Read the model definition and answer for the solid it produces. Units are mm, in the model's axes. A direction names the side the tool comes from. Round coordinates to 2 decimals unless told otherwise and drop trailing zeros. Order: outer loops, then holes, each group sorted by start corner. A loop starts at its lowest first (then second) coordinate and runs counter-clockwise, first axis right, second up. Notation, with made-up numbers: (57, 32) -> (102, 32) arc R27 cw to (102, 69) -> close; hole circle Ø10 at (56, 27.5). An arc over 180 degrees is marked (long way). One line per item, written item: value. Start each with the question number.
1. For faces 5 (the face through (-431, 6.75, 620)), 6 (the face through (-3, 358.24, -9)), 7 (the face through (430, 8.25, -620)), 8 (the face through (305.38, 178.55, -8.86)), 9 (the face through (-430, 8.25, 620)), determine the directions among +Z, -Z, +X, -X, +Y, -Y from which every point of the face is accessible in a straight line to the end or side of a thin tool.
2. Section B-B (y = 283.5) is taken. Give the vertices of the cut face in (x, z), then the cut area to 3 significant figures.
3. Section D-D (x = -354) is taken. Give the vertices of the cut face in (y, z), then the cut area to 3 significant figures.
4. Section A-A (z = 13) is taken. Give the vertices of the cut face in (x, y), then the cut area to 3 significant figures.
5. Flat-ended cylindrical pins translate along their axes: pin 1 Ø10.5 at (x, z) = (427, -615) entering from +Y; pin 2 Ø4 at (x, z) = (-204, 104) entering from -Y; pin 3 Ø3 at (y, z) = (290.5, -207.5) entering from +X. Find the tip coordinate at first contact, or state that the pin passes through.
6. The mould has two halves that part along X. Classify faces 1 (the face through (431, 6.75, 620)), 2 (the face through (303.85, 184.2, -8.86)), 3 (the face through (-302.55, 183.45, -8.86)), 4 (the face through (3, 356.74, -9)): released by +X, released by -X, zero draft, split by the parting line, or undercut.
7. Section C-C (x = 1.5) is taken. Give the vertices of the cut face in (y, z).
8. Consider line 1 (Z direction, x = -447, y = 7); line 2 (X direction, y = 7, z = -615); line 3 (X direction, y = 7.65, z = -615). Determine where each line is inside the solid, lowest interval first.
from build123d import *

# Parameters (mm, degrees)
EXTRUDE_1_DEPTH          = 633
EXTRUDE_1_DEPTH_BACK     = 633
SHEET_START              = -633
SHEET_METAL_1_DEPTH      = 1266
SHEET_METAL_1_2_DEPTH    = 1266
SM_START                 = -633
SM_EDGE_FLANGE_1_DEPTH   = 33.75
SM_START_2               = -600
SM_EDGE_FLANGE_1_2_DEPTH = 0.75
SM_EDGE_FLANGE_1_3_DEPTH = 33
MIRROR_START             = -633
MIRROR_2_COPY_1_DEPTH    = 33.75
MIRROR_START_2           = -600
MIRROR_2_COPY_2_DEPTH    = 0.75
MIRROR_2_COPY_3_DEPTH    = 33
MIRROR_2_COPY_4_DEPTH    = 0.75
MIRROR_2_COPY_5_DEPTH    = 33
CUT_EXTRUDE_1_REACH      = 856.061
SKETCH_9_R               = 4


# Read off the part's stored shape, not the designer's step: Преобразовать-Твердое тело1, Ребро-кромка1
with BuildPart() as part:
    # Sketch 1 → Вытянуть-Тонкостенный1 (new, two sides: drawn at the far end of the back side and taken through both)
    with BuildSketch(Plane.XY.offset(-EXTRUDE_1_DEPTH_BACK)):
        Polygon((405, 6), (202.5, 356.740288533), (-202.5, 356.740288533), (-405, 6), (-406.299038106, 6.75), (-203.366025404, 358.240288533), (203.366025404, 358.240288533), (406.299038106, 6.75), align=None)
    extrude(amount=EXTRUDE_1_DEPTH + EXTRUDE_1_DEPTH_BACK)

    # Sheet Metal 1 outline → Sheet Metal 1 (cut)
    with BuildSketch(Plane.XY.offset(SHEET_START)):
        with BuildLine():
            Line((203.366025404, 358.240288533), (201.633974596, 358.240288533))
            ThreePointArc((201.633974596, 358.240288533), (203.133974596, 357.838364744), (204.232050808, 356.740288533))
            Line((204.232050808, 356.740288533), (203.366025404, 358.240288533))
        make_face()
        with BuildLine():
            ThreePointArc((-204.232050808, 356.740288533), (-203.133974596, 357.838364744), (-201.633974596, 358.240288533))
            Line((-201.633974596, 358.240288533), (-203.366025404, 358.240288533))
            Line((-203.366025404, 358.240288533), (-204.232050808, 356.740288533))
        make_face()
    extrude(amount=SHEET_METAL_1_DEPTH, mode=Mode.SUBTRACT)

    # Sheet Metal 1 2 outline → Sheet Metal 1 2 (add)
    with BuildSketch(Plane.XY.offset(SHEET_START)):
        with BuildLine():
            Line((202.5, 356.740288533), (201.633974596, 356.740288533))
            ThreePointArc((201.633974596, 356.740288533), (202.383974596, 356.539326638), (202.933012702, 355.990288533))
            Line((202.933012702, 355.990288533), (202.5, 356.740288533))
        make_face()
        with BuildLine():
            ThreePointArc((-202.933012702, 355.990288533), (-202.383974596, 356.539326638), (-201.633974596, 356.740288533))
            Line((-201.633974596, 356.740288533), (-202.5, 356.740288533))
            Line((-202.5, 356.740288533), (-202.933012702, 355.990288533))
        make_face()
    extrude(amount=SHEET_METAL_1_2_DEPTH)

    # Ребро-кромка1 outline → Ребро-кромка1 (cut)
    with BuildSketch(Plane.XY.offset(SM_START)):
        with BuildLine():
            Line((-405, 6), (-403.700961894, 8.25))
            ThreePointArc((-403.700961894, 8.25), (-404.799038106, 7.151923789), (-406.299038106, 6.75))
            Line((-406.299038106, 6.75), (-405, 6))
        make_face()
    sm_edge_flange_1 = extrude(amount=SM_EDGE_FLANGE_1_DEPTH, mode=Mode.SUBTRACT)

    # Sm Edge Flange 1 2 outline → Sm Edge Flange 1 2 (cut)
    with BuildSketch(Plane.XY.offset(SM_START_2)):
        with BuildLine():
            Line((-403.325961894, 8.899519053), (-404.625, 9.649519053))
            Line((-404.625, 9.649519053), (-406.299038106, 6.75))
            ThreePointArc((-406.299038106, 6.75), (-404.799038106, 7.151923789), (-403.700961894, 8.25))
            Line((-403.700961894, 8.25), (-403.325961894, 8.899519053))
        make_face()
    sm_edge_flange_1_2 = extrude(amount=SM_EDGE_FLANGE_1_2_DEPTH, mode=Mode.SUBTRACT)

    # Sm Edge Flange 1 3 outline → Sm Edge Flange 1 3 (add)
    with BuildSketch(Plane.XY.offset(SM_START)):
        with BuildLine():
            Line((-406.299038106, 6.75), (-405, 9))
            ThreePointArc((-405, 9), (-405.549038106, 8.450961894), (-406.299038106, 8.25))
            Line((-406.299038106, 8.25), (-454.133974596, 8.25))
            Line((-454.133974596, 8.25), (-454.133974596, 6.75))
            Line((-454.133974596, 6.75), (-406.299038106, 6.75))
        make_face()
    sm_edge_flange_1_3 = extrude(amount=SM_EDGE_FLANGE_1_3_DEPTH)

    # Зеркальное отражение1: Ребро-кромка1, Sm Edge Flange 1 2, Sm Edge Flange 1 3 across plane
    add(sm_edge_flange_1.mirror(Plane.XY), mode=Mode.SUBTRACT)
    add(sm_edge_flange_1_2.mirror(Plane.XY), mode=Mode.SUBTRACT)
    add(sm_edge_flange_1_3.mirror(Plane.XY))

    # Зеркальное отражение2: Ребро-кромка1, Sm Edge Flange 1 2, Sm Edge Flange 1 3 across plane
    add(sm_edge_flange_1.mirror(Plane(origin=(0, 0, 0), x_dir=(0, 0, 1), z_dir=(1, 0, 0))), mode=Mode.SUBTRACT)
    add(sm_edge_flange_1_2.mirror(Plane(origin=(0, 0, 0), x_dir=(0, 0, 1), z_dir=(1, 0, 0))), mode=Mode.SUBTRACT)
    add(sm_edge_flange_1_3.mirror(Plane(origin=(0, 0, 0), x_dir=(0, 0, 1), z_dir=(1, 0, 0))))

    # Зеркальное отражение2 copy 1 sketch → Зеркальное отражение2 copy 1 (cut)
    with BuildSketch(Plane(origin=(0, 0, 0), x_dir=(-1, 0, 0), z_dir=(0, 0, -1)).offset(MIRROR_START)):
        with BuildLine():
            Line((-405, 6), (-403.700961894, 8.25))
            ThreePointArc((-403.700961894, 8.25), (-404.799038106, 7.151923789), (-406.299038106, 6.75))
            Line((-406.299038106, 6.75), (-405, 6))
        make_face()
    extrude(amount=MIRROR_2_COPY_1_DEPTH, mode=Mode.SUBTRACT)

    # Зеркальное отражение2 copy 2 sketch → Зеркальное отражение2 copy 2 (cut)
    with BuildSketch(Plane(origin=(0, 0, 0), x_dir=(-1, 0, 0), z_dir=(0, 0, -1)).offset(MIRROR_START_2)):
        with BuildLine():
            Line((-403.325961894, 8.899519053), (-404.625, 9.649519053))
            Line((-404.625, 9.649519053), (-406.299038106, 6.75))
            ThreePointArc((-406.299038106, 6.75), (-404.799038106, 7.151923789), (-403.700961894, 8.25))
            Line((-403.700961894, 8.25), (-403.325961894, 8.899519053))
        make_face()
    extrude(amount=MIRROR_2_COPY_2_DEPTH, mode=Mode.SUBTRACT)

    # Зеркальное отражение2 copy 3 sketch → Зеркальное отражение2 copy 3 (add)
    with BuildSketch(Plane(origin=(0, 0, 0), x_dir=(-1, 0, 0), z_dir=(0, 0, -1)).offset(MIRROR_START)):
        with BuildLine():
            Line((-406.299038106, 6.75), (-405, 9))
            ThreePointArc((-405, 9), (-405.549038106, 8.450961894), (-406.299038106, 8.25))
            Line((-406.299038106, 8.25), (-454.133974596, 8.25))
            Line((-454.133974596, 8.25), (-454.133974596, 6.75))
            Line((-454.133974596, 6.75), (-406.299038106, 6.75))
        make_face()
    extrude(amount=MIRROR_2_COPY_3_DEPTH)

    # Зеркальное отражение2 copy 4 sketch → Зеркальное отражение2 copy 4 (cut)
    with BuildSketch(Plane(origin=(0, 0, 0), x_dir=(-1, 0, 0), z_dir=(0, 0, 1)).offset(MIRROR_START_2)):
        with BuildLine():
            Line((-403.325961894, -8.899519053), (-404.625, -9.649519053))
            Line((-404.625, -9.649519053), (-406.299038106, -6.75))
            ThreePointArc((-406.299038106, -6.75), (-404.799038106, -7.151923789), (-403.700961894, -8.25))
            Line((-403.700961894, -8.25), (-403.325961894, -8.899519053))
        make_face()
    extrude(amount=MIRROR_2_COPY_4_DEPTH, mode=Mode.SUBTRACT)

    # Зеркальное отражение2 copy 5 sketch → Зеркальное отражение2 copy 5 (add)
    with BuildSketch(Plane(origin=(0, 0, 0), x_dir=(-1, 0, 0), z_dir=(0, 0, 1)).offset(MIRROR_START)):
        with BuildLine():
            Line((-406.299038106, -6.75), (-405, -9))
            ThreePointArc((-405, -9), (-405.549038106, -8.450961894), (-406.299038106, -8.25))
            Line((-406.299038106, -8.25), (-454.133974596, -8.25))
            Line((-454.133974596, -8.25), (-454.133974596, -6.75))
            Line((-454.133974596, -6.75), (-406.299038106, -6.75))
        make_face()
    extrude(amount=MIRROR_2_COPY_5_DEPTH)

    # Эскиз9 → Вырез-Вытянуть1 (cut, up to next)
    with BuildSketch(Plane(origin=(0, 8.25, 0), x_dir=(1, 0, 0), z_dir=(0, 1, 0)), mode=Mode.PRIVATE) as cut_extrude_1_sk1:
        with Locations(Location((-447, 615, 0), (0, 0, 180))):
            Circle(SKETCH_9_R)
    cut_extrude_1_tool1 = extrude(cut_extrude_1_sk1.sketch, amount=-CUT_EXTRUDE_1_REACH, mode=Mode.PRIVATE) & part.part
    # Эскиз9 → Вырез-Вытянуть1 (cut, up to next)
    with BuildSketch(Plane(origin=(0, 8.25, 0), x_dir=(1, 0, 0), z_dir=(0, 1, 0)), mode=Mode.PRIVATE) as cut_extrude_1_sk2:
        with Locations(Location((-427, 615, 0), (0, 0, 180))):
            Circle(SKETCH_9_R)
    cut_extrude_1_tool2 = extrude(cut_extrude_1_sk2.sketch, amount=-CUT_EXTRUDE_1_REACH, mode=Mode.PRIVATE) & part.part
    # Эскиз9 → Вырез-Вытянуть1 (cut, up to next)
    with BuildSketch(Plane(origin=(0, 8.25, 0), x_dir=(1, 0, 0), z_dir=(0, 1, 0)), mode=Mode.PRIVATE) as cut_extrude_1_sk3:
        with Locations(Location((-447, -615, 0), (0, 0, 180))):
            Circle(SKETCH_9_R)
    cut_extrude_1_tool3 = extrude(cut_extrude_1_sk3.sketch, amount=-CUT_EXTRUDE_1_REACH, mode=Mode.PRIVATE) & part.part
    # Эскиз9 → Вырез-Вытянуть1 (cut, up to next)
    with BuildSketch(Plane(origin=(0, 8.25, 0), x_dir=(1, 0, 0), z_dir=(0, 1, 0)), mode=Mode.PRIVATE) as cut_extrude_1_sk4:
        with Locations(Location((-427, -615, 0), (0, 0, 180))):
            Circle(SKETCH_9_R)
    cut_extrude_1_tool4 = extrude(cut_extrude_1_sk4.sketch, amount=-CUT_EXTRUDE_1_REACH, mode=Mode.PRIVATE) & part.part
    # Эскиз9 → Вырез-Вытянуть1 (cut, up to next)
    with BuildSketch(Plane(origin=(0, 8.25, 0), x_dir=(1, 0, 0), z_dir=(0, 1, 0)), mode=Mode.PRIVATE) as cut_extrude_1_sk5:
        with Locations(Location((427, -615, 0), (0, 0, 180))):
            Circle(SKETCH_9_R)
    cut_extrude_1_tool5 = extrude(cut_extrude_1_sk5.sketch, amount=-CUT_EXTRUDE_1_REACH, mode=Mode.PRIVATE) & part.part
    # Эскиз9 → Вырез-Вытянуть1 (cut, up to next)
    with BuildSketch(Plane(origin=(0, 8.25, 0), x_dir=(1, 0, 0), z_dir=(0, 1, 0)), mode=Mode.PRIVATE) as cut_extrude_1_sk6:
        with Locations(Location((447, -615, 0), (0, 0, 180))):
            Circle(SKETCH_9_R)
    cut_extrude_1_tool6 = extrude(cut_extrude_1_sk6.sketch, amount=-CUT_EXTRUDE_1_REACH, mode=Mode.PRIVATE) & part.part
    # Эскиз9 → Вырез-Вытянуть1 (cut, up to next)
    with BuildSketch(Plane(origin=(0, 8.25, 0), x_dir=(1, 0, 0), z_dir=(0, 1, 0)), mode=Mode.PRIVATE) as cut_extrude_1_sk7:
        with Locations(Location((427, 615, 0), (0, 0, 180))):
            Circle(SKETCH_9_R)
    cut_extrude_1_tool7 = extrude(cut_extrude_1_sk7.sketch, amount=-CUT_EXTRUDE_1_REACH, mode=Mode.PRIVATE) & part.part
    # Эскиз9 → Вырез-Вытянуть1 (cut, up to next)
    with BuildSketch(Plane(origin=(0, 8.25, 0), x_dir=(1, 0, 0), z_dir=(0, 1, 0)), mode=Mode.PRIVATE) as cut_extrude_1_sk8:
        with Locations(Location((447, 615, 0), (0, 0, 180))):
            Circle(SKETCH_9_R)
    cut_extrude_1_tool8 = extrude(cut_extrude_1_sk8.sketch, amount=-CUT_EXTRUDE_1_REACH, mode=Mode.PRIVATE) & part.part
    add(cut_extrude_1_tool1.solids().sort_by_distance((-447, 8.25, -615))[0], mode=Mode.SUBTRACT)
    add(cut_extrude_1_tool2.solids().sort_by_distance((-427, 8.25, -615))[0], mode=Mode.SUBTRACT)
    add(cut_extrude_1_tool3.solids().sort_by_distance((-447, 8.25, 615))[0], mode=Mode.SUBTRACT)
    add(cut_extrude_1_tool4.solids().sort_by_distance((-427, 8.25, 615))[0], mode=Mode.SUBTRACT)
    add(cut_extrude_1_tool5.solids().sort_by_distance((427, 8.25, 615))[0], mode=Mode.SUBTRACT)
    add(cut_extrude_1_tool6.solids().sort_by_distance((447, 8.25, 615))[0], mode=Mode.SUBTRACT)
    add(cut_extrude_1_tool7.solids().sort_by_distance((427, 8.25, -615))[0], mode=Mode.SUBTRACT)
    add(cut_extrude_1_tool8.solids().sort_by_distance((447, 8.25, -615))[0], mode=Mode.SUBTRACT)


solid = part.part
Answer:
1. face 5: +Z, -Z, +X, -X, -Y
1. face 6: +Z, -Z, +X, -X, +Y
1. face 7: +Z, -Z, +X, +Y
1. face 8: +Z, -Z, -Y
1. face 9: +Z, -Z, -X, +Y
2. outline: (-246.52, -633) -> (-244.79, -633) -> (-244.79, 633) -> (-246.52, 633) -> close; (244.79, -633) -> (246.52, -633) -> (246.52, 633) -> (244.79, 633) -> close
2. area: 4,390 mm^2
3. outline: (94.33, -633) -> (97.33, -633) -> (97.33, 633) -> (94.33, 633) -> close
3. area: 3,800 mm^2
4. outline: (-406.3, 6.75) -> (-405, 6) -> (-202.93, 355.99) arc R1.5 cw to (-201.63, 356.74) -> (201.63, 356.74) arc R1.5 cw to (202.93, 355.99) -> (405, 6) -> (406.3, 6.75) -> (204.23, 356.74) arc R3 ccw to (201.63, 358.24) -> (-201.63, 358.24) arc R3 ccw to (-204.23, 356.74) -> close
4. area: 1,820 mm^2
5. pin 1: y = 8.25
5. pin 2: y = 350.68
5. pin 3: x = 243.34
6. face 1: zero draft
6. face 2: released by +X
6. face 3: undercut
6. face 4: undercut
7. outline: (356.74, -633) -> (358.24, -633) -> (358.24, 633) -> (356.74, 633) -> close
8. line 1: -633 to -619, -611 to -600, 600 to 611, 619 to 633
8. line 2: -454.13 to -451, -443 to -431, -423 to -405.1, 405.1 to 423, 431 to 443, 451 to 454.13
8. line 3: -454.13 to -451, -443 to -431, -423 to -404.16, 404.16 to 423, 431 to 443, 451 to 454.13
